```python
from build123d import *

# Parameters (mm, degrees)
BOSS_EXTRUDE1_DEPTH = 6
BOSS_EXTRUDE2_DEPTH = 1.5
FILLET6_R           = 0.05


with BuildPart() as part:
    # Sketch2 → Boss-Extrude1 (new body)
    with BuildSketch(Plane.XY):
        Polygon((-0.8, 2.7), (0.8, 2.7), (0.8, 1.3), (1.8, 1.3), (1.8, 0), (-1.8, 0), (-1.8, 1.3), (-0.8, 1.3), align=None)
    extrude(amount=BOSS_EXTRUDE1_DEPTH)

    # Sketch3 → Boss-Extrude2 (add)
    with BuildSketch(Plane(origin=(0, 2.7, 0), x_dir=(1, 0, 0), z_dir=(0, 1, 0))):
        with BuildLine():
            ThreePointArc((0.8, -0.108633541), (0, 0), (-0.8, -0.108633541))
            Line((-0.8, -0.108633541), (-0.8, -5.891366459))
            ThreePointArc((-0.8, -5.891366459), (0, -6), (0.8, -5.891366459))
            Line((0.8, -5.891366459), (0.8, -0.108633541))
        make_face()
        with BuildLine():
            Line((-2.828427125, -2), (-1, -2))
            Line((-1, -2), (-1, -4))
            Line((-1, -4), (-2.828427125, -4))
            ThreePointArc((-2.828427125, -4), (-2.04589531, -5.194154138), (-0.8, -5.891366459))
            Line((-0.8, -5.891366459), (-0.8, -0.108633541))
            ThreePointArc((-0.8, -0.108633541), (-2.04589531, -0.805845862), (-2.828427125, -2))
        make_face()
        with BuildLine():
            ThreePointArc((2.828427125, -2), (2.04589531, -0.805845862), (0.8, -0.108633541))
            Line((0.8, -0.108633541), (0.8, -5.891366459))
            ThreePointArc((0.8, -5.891366459), (2.04589531, -5.194154138), (2.828427125, -4))
            Line((2.828427125, -4), (1, -4))
            Line((1, -4), (1, -2))
            Line((1, -2), (2.828427125, -2))
        make_face()
    extrude(amount=BOSS_EXTRUDE2_DEPTH)

    # Fillet6
    fillet6_edges = [part.edges().sort_by_distance(p)[0] for p in [
        (0.8, 1.3, 3),
        (1.8, 1.3, 3),
        (-1.8, 1.3, 3),
        (-0.8, 1.3, 3),
    ]]
    fillet(fillet6_edges, radius=FILLET6_R)


solid = part.part
```
Can you work these out from the model? Positions are in its coordinate system, mm. A direction names the side the tool comes from. Coordinates: 2 decimals unless noted, no trailing zeros. Loops run counter-clockwise (first coordinate to the right, second up) from the corner with the lowest first, then second, coordinate; pieces in that order, holes last.
1) Imagine slicing it at A-A on y = 3.1. List the corners of the cut face in (x, z) for me, plus the area to 3 significant figures.
2) Imagine slicing it at C-C on z = 2.2. List the corners of the cut face in (x, y) for me, plus the area to 3 significant figures.
3) Which directions (+Z, -Z, +X, -X, +Y, -Y) give clear straight access to the entire face, cutting with the end or side of a thin tool? Please do faces 1 (the flat face through (-1.6, 2.7, 4.2)), 2 (the flat face through (-1, 3, 3)), 3 (the flat face through (1.8, 1, 3)), 4 (the flat face through (-1.8, 1, 3)), 5 (the flat face through (0.8, 2, 3)).
4) Imagine slicing it at B-B on x = 1.2. List the corners of the cut face in (y, z) for me, plus the area to 3 significant figures.
5) I need wall thicknesses on probe 1 along Y at (x, z) = (1.65, 0.95); probe 2 along X at (y, z) = (3.3, 3.65); probe 3 along X at (y, z) = (2, 3.7). Which ranges of each line are inside material? Lowest first, please.
6) For pin 1 (1.6 mm diameter, centred on y = 3.5, z = 3, fed in from -X); pin 2 (2 mm diameter, centred on y = 1, z = 2.5, fed in from +X); pin 3 (0.6 mm diameter, centred on y = 0.5, z = 3.5, fed in from -X), each with a flat end and sliding along its axis, tell me the tip position at first contact or that it passes through.
7) Imagine slicing it at D-D on x = -1.35. List the corners of the cut face in (y, z) for me.
8) Thinking about a two-plate mould opening in Z: for faces 6 (the flat face through (-2, 3, 2)), 7 (the flat face through (0, 1, 0)), 8 (the flat face through (1.3, 1.3, 3)), 9 (the flat face through (2, 3, 2)), which applies, pulls with the +Z half, pulls with the -Z half, needs draft (parallel to the pull), parting line crosses it, or undercut?
Completed:
1. outline: (-2.83, 2) arc R3 ccw to (2.83, 2) - (1, 2) - (1, 4) - (2.83, 4) arc R3 ccw to (-2.83, 4) - (-1, 4) - (-1, 2) - close
1. area: 20.5 mm2
2. outline: (-1.8, 0) - (1.8, 0) - (1.8, 1.25) arc R0.05 ccw to (1.75, 1.3) - (0.85, 1.3) arc R0.05 cw to (0.8, 1.35) - (0.8, 2.7) - (1, 2.7) - (1, 4.2) - (-1, 4.2) - (-1, 2.7) - (-0.8, 2.7) - (-0.8, 1.35) arc R0.05 cw to (-0.85, 1.3) - (-1.75, 1.3) arc R0.05 ccw to (-1.8, 1.25) - close
2. area: 9.92 mm2
3. face 1: +Z, -Z, -X
3. face 2: -X, +Y
3. face 3: +Z, -Z, +X, -Y
3. face 4: +Z, -Z, -X, -Y
3. face 5: +Z, -Z, +X
4. outline: (0, 0) - (1.3, 0) - (1.3, 6) - (0, 6) - close; (2.7, 0.25) - (4.2, 0.25) - (4.2, 2) - (2.7, 2) - close; (2.7, 4) - (4.2, 4) - (4.2, 5.75) - (2.7, 5.75) - close
4. area: 13.0 mm2
5. probe 1: y = 0 to 1.3, 2.7 to 4.2
5. probe 2: x = -1 to 1
5. probe 3: x = -0.8 to 0.8
6. pin 1: stops at x = -1
6. pin 2: stops at x = 1.8
6. pin 3: stops at x = -1.8
7. outline: (0, 0) - (1.3, 0) - (1.3, 6) - (0, 6) - close; (2.7, 0.32) - (4.2, 0.32) - (4.2, 2) - (2.7, 2) - close; (2.7, 4) - (4.2, 4) - (4.2, 5.68) - (2.7, 5.68) - close
8. face 6: undercut
8. face 7: pulls with the -Z half
8. face 8: needs draft
8. face 9: undercut
